Job drawing, mm, ordinate dimensions from the low corner. One solid piece. A direction names the side the tool comes from. Coordinates: 2 decimals unless noted, no trailing zeros. Loops run counter-clockwise (first coordinate to the right, second up) from the corner with the lowest first, then second, coordinate; pieces in that order, holes last. Notation, with made-up numbers: M -2.75,14 L 34.25,14 A8 cw 34.25,29 Z; hole C 13,7 d10. An arc over 180 degrees is marked long. Answer as a JSON object with one key per item and string values. Group by question number.
1. Mould opens along Y. For the marked faces 1, 2 and 3 say: released by +Y, released by -Y, zero draft, split by the parting line, or undercut.
2. Drop flat-ended pins along their axis: pin 1 Ø1 at (x, y) = (51, 10.5) entering from +Z; pin 2 Ø3 at (x, y) = (49, 6) entering from -Z; pin 3 Ø6 at (y, z) = (13, 66) entering from -X; pin 4 Ø10 at (x, z) = (17.5, 40.5) entering from -Y. Give the stop position or say it passes through.
3. Drill centre lines: L1, parallel to Z at x = 38.1, y = 16.25 (1 decimal); L2, parallel to Z at x = 38.1, y = 18 (1 decimal); L3, parallel to Y at x = 57.5, z = 16. Where is each one in solid material? Low to high.
4. 3-axis set-ups, long thin cutter, end or side, ignore diameter. For the marked faces 4 and 5: which of +Z, -Z, +X, -X, +Y, -Y reach the whole face in a straight line?
5. Saw through at C-C on x = 19. Write the cut outline in (y, z).
6. Saw through at A-A on z = 38.1. Write the cut outline in (x, y) (1 decimal), then the cut area to 3 significant figures.
7. Saw through at B-B on x = 38.1. Write the cut outline in (y, z) (1 decimal), then the cut area to 3 significant figures.
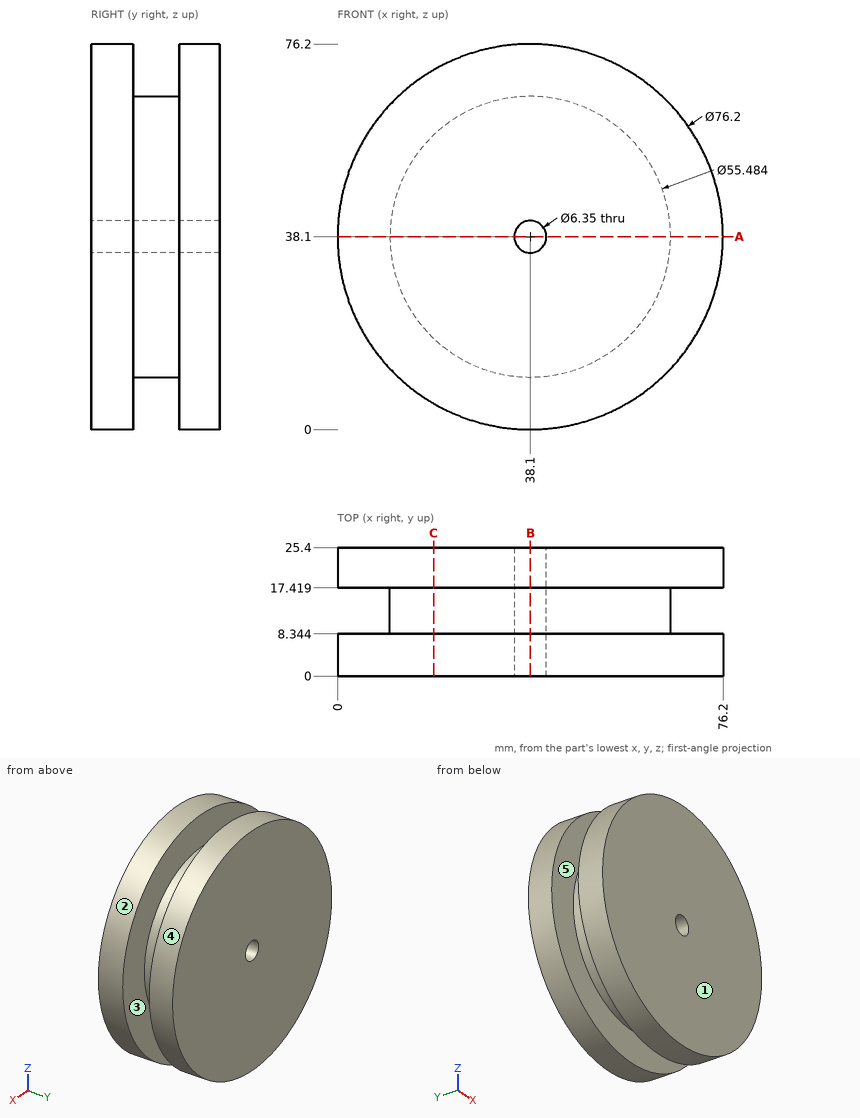
Outcome:
{
 "1": {"face 1": "released by -Y", "face 2": "zero draft", "face 3": "undercut"},
 "2": {"pin 1": "stops at z = 62.92", "pin 2": "stops at z = 1.18", "pin 3": "stops at x = 25.87", "pin 4": "stops at y = 0"},
 "3": {"L1": "z = 10.4 to 34.9, 41.3 to 65.8", "L2": "z = 0 to 34.9, 41.3 to 76.2", "L3": "y = 0 to 8.34, 17.42 to 25.4"},
 "4": {"face 4": "+Y, -Y", "face 5": "none"},
 "5": {"outline": "M 0,5.13 L 8.34,5.13 L 8.34,17.98 L 17.42,17.98 L 17.42,5.13 L 25.4,5.13 L 25.4,71.07 L 17.42,71.07 L 17.42,58.22 L 8.34,58.22 L 8.34,71.07 L 0,71.07 Z"},
 "6": {"outline": "M 0,0 L 34.9,0 L 34.9,25.4 L 0,25.4 L 0,17.4 L 10.4,17.4 L 10.4,8.3 L 0,8.3 Z; M 41.3,0 L 76.2,0 L 76.2,8.3 L 65.8,8.3 L 65.8,17.4 L 76.2,17.4 L 76.2,25.4 L 41.3,25.4 Z", "area": "1,590 mm²"},
 "7": {"outline": "M 0,0 L 8.3,0 L 8.3,10.4 L 17.4,10.4 L 17.4,0 L 25.4,0 L 25.4,34.9 L 0,34.9 Z; M 0,41.3 L 25.4,41.3 L 25.4,76.2 L 17.4,76.2 L 17.4,65.8 L 8.3,65.8 L 8.3,76.2 L 0,76.2 Z", "area": "1,590 mm²"}
}
